```python
from build123d import *

# Parameters (mm, degrees)
SKETCH2_R           = 15
BOSS_EXTRUDE1_DEPTH = 162
SKETCH3_W           = 75
SKETCH3_H           = 106
CUT_EXTRUDE1_DEPTH  = 200.03014847
SKETCH4_R           = 44
SKETCH4_R_2         = 25
BOSS_EXTRUDE2_DEPTH = 70
CUT_EXTRUDE5_START  = -60
CUT_EXTRUDE5_DEPTH  = 60
SCALE1_SCALE        = 0.33


with BuildPart() as part:
    # Sketch2 → Boss-Extrude1 (new body)
    with BuildSketch(Plane.XY):
        with BuildLine():
            Line((-75, -44), (-45, -44))
            Line((-45, -44), (8.212754936, -28.853953912))
            ThreePointArc((8.212754936, -28.853953912), (30, 0), (8.212754936, 28.853953912))
            Line((8.212754936, 28.853953912), (-45, 44))
            Line((-45, 44), (-75, 44))
            Line((-75, 44), (-75, -44))
        make_face()
        Circle(SKETCH2_R, mode=Mode.SUBTRACT)
    extrude(amount=BOSS_EXTRUDE1_DEPTH)

    # Sketch3 → Cut-Extrude1 (cut, through all)
    with BuildSketch(Plane.XZ.offset(44)):
        with Locations((-7.5, 81)):
            Rectangle(SKETCH3_W, SKETCH3_H)
    extrude(amount=-CUT_EXTRUDE1_DEPTH, mode=Mode.SUBTRACT)

    # Sketch4 → Boss-Extrude2 (add)
    with BuildSketch(Plane.ZY.offset(75)):
        with Locations(Location((81, 0, 0), (0, 0, 270))):
            Circle(SKETCH4_R)
        with Locations(Location((81, 0, 0), (0, 0, 270))):
            Circle(SKETCH4_R_2, mode=Mode.SUBTRACT)
    extrude(amount=BOSS_EXTRUDE2_DEPTH)

    # Sketch7 → Cut-Extrude5 (cut)
    with BuildSketch(Plane.ZY.offset(145).offset(CUT_EXTRUDE5_START)):
        with BuildLine():
            Line((50.06906521, -4), (56.322074641, -4))
            ThreePointArc((56.322074641, -4), (56, 0), (56.322074641, 4))
            Line((56.322074641, 4), (50.06906521, 4))
            Line((50.06906521, 4), (50.06906521, -4))
        make_face()
    extrude(amount=CUT_EXTRUDE5_DEPTH, mode=Mode.SUBTRACT)


with BuildPart() as part_1:
    # Scale1: scaled about (-64.229382242, 0, 81.085826585)
    add(part.part.scale(SCALE1_SCALE).moved(Location((-43.033686102, 0, 54.327503812))))


solid = part_1.part
```
Here's how the part is built. I have some questions about the finished solid (model axes, mm). A direction names the side the tool comes from. Coordinates: 2 decimals unless noted, no trailing zeros. Order: outer loops, then holes, each group sorted by start corner. A loop starts at its lowest first (then second) coordinate and runs counter-clockwise, first axis right, second up.
1) We'd pull the mould along Y, two halves only. Please class faces 4 (the face through (-48.4, -0.2, 63.568)), 5 (the face through (-81, -1.32, 72)), 6 (the face through (-33.135, -0.179, 103.103)): +Y half, -Y half, draft (parallel to the pull), parting line (faces both ways), or undercut.
2) Imagine slicing it at C-C on y = 11.5. List the corners of the cut face in (x, z) for me, and give its area (3 significant figures).
3) Imagine slicing it at B-B on z = 78. List the corners of the cut face in (x, y) for me, and give its area (3 significant figures).
4) Which directions (+Z, -Z, +X, -X, +Y, -Y) give clear straight access to the entire face, cutting with the end or side of a thin tool? Please do faces 1 (the face through (-33.135, -0.179, 58.883)), 2 (the face through (-48.4, -0.2, 98.548)), 3 (the face through (-81, 0, 70.85)).
5) I need wall thicknesses on line 1 (X direction, y = 0, z = 105.25); line 2 (Z direction, x = -51, y = 2.5); line 3 (Z direction, x = -86, y = 0). Which ranges of each line are inside material? Lowest first, please.
6) Imagine slicing it at D-D on y = -3.25. List the corners of the cut face in (x, z) for me, and give its area (3 significant figures).
7) Imagine slicing it at A-A on y = 0. List the corners of the cut face in (x, z) for me.
8) Will these pins go through, and if not, where does the flat tip stop? pin 1 (0.8 mm diameter, centred on x = -77, y = 0.5, fed in from +Z); pin 2 (1 mm diameter, centred on x = -85, z = 72.5, fed in from +Y); pin 3 (10 mm diameter, centred on y = 0, z = 81.06, fed in from -X).
Response values:
1. face 4: draft
1. face 5: undercut
1. face 6: parting line
2. outline: (-90.88, 72.19) - (-67.78, 72.19) - (-67.78, 54.33) - (-47.27, 54.33) - (-47.27, 63.57) - (-57.88, 63.57) - (-57.88, 98.55) - (-47.27, 98.55) - (-47.27, 107.79) - (-67.78, 107.79) - (-67.78, 89.92) - (-90.88, 89.92) - close
2. area: 1,130 mm2
3. outline: (-90.88, -14.19) - (-67.78, -14.19) - (-67.78, -14.52) - (-57.88, -14.52) - (-57.88, 14.52) - (-67.78, 14.52) - (-67.78, 14.19) - (-90.88, 14.19) - (-90.88, 7.66) - (-67.78, 7.66) - (-67.78, -7.66) - (-90.88, -7.66) - close
3. area: 589 mm2
4. face 1: +Z, -Z, +X
4. face 2: +X, +Y, -Y
4. face 3: -X
5. line 1: x = -67.78 to -47.98, -38.08 to -33.13
5. line 2: z = 54.33 to 63.57, 98.55 to 107.79
5. line 3: z = 66.54 to 70.85, 89.31 to 95.58
6. outline: (-90.88, 66.91) - (-67.78, 66.91) - (-67.78, 54.33) - (-46.77, 54.33) - (-46.77, 63.57) - (-57.88, 63.57) - (-57.88, 98.55) - (-46.77, 98.55) - (-46.77, 107.79) - (-67.78, 107.79) - (-67.78, 95.21) - (-90.88, 95.21) - (-90.88, 88.64) - (-67.78, 88.64) - (-67.78, 73.47) - (-90.88, 73.47) - close; (-39.3, 54.33) - (-33.68, 54.33) - (-33.68, 63.57) - (-39.3, 63.57) - close; (-39.3, 98.55) - (-33.68, 98.55) - (-33.68, 107.79) - (-39.3, 107.79) - close
6. area: 1,140 mm2
7. outline: (-90.88, 66.54) - (-67.78, 66.54) - (-67.78, 54.33) - (-47.98, 54.33) - (-47.98, 63.57) - (-57.88, 63.57) - (-57.88, 98.55) - (-47.98, 98.55) - (-47.98, 107.79) - (-67.78, 107.79) - (-67.78, 95.58) - (-90.88, 95.58) - (-90.88, 89.31) - (-67.78, 89.31) - (-67.78, 72.81) - (-71.08, 72.81) - (-71.08, 70.85) - (-90.88, 70.85) - close; (-38.08, 54.33) - (-33.13, 54.33) - (-33.13, 63.57) - (-38.08, 63.57) - close; (-38.08, 98.55) - (-33.13, 98.55) - (-33.13, 107.79) - (-38.08, 107.79) - close
8. pin 1: stops at z = 95.58
8. pin 2: stops at y = 12.08
8. pin 3: stops at x = -67.78
